Model file for the job. Use its own axes, mm. A direction names the side the tool comes from. Round coordinates to 2 decimals unless told otherwise and drop trailing zeros. Loops run counter-clockwise (first coordinate to the right, second up) from the corner with the lowest first, then second, coordinate; pieces in that order, holes last. Notation, with made-up numbers: (46.25, -2.75) - (99.25, -2.75) arc R24 ccw to (99.25, 24.25) - close; hole circle Ø1 at (60.25, 84). An arc over 180 degrees is marked (long way). Answer as a JSON object with one key per item and string values.
from build123d import *

# Parameters (mm, degrees)
ESQUISSE1_R                  = 18
BOSS_EXTRU_1_DEPTH           = 4
ESQUISSE5_R                  = 25.5
BOSS_EXTRU_2_DEPTH           = 0.6
ENL_V_MAT_EXTRU_1_DEPTH      = 37.354642069
ESQUISSE4_R                  = 4
ENL_V_MAT_EXTRU_3_DEPTH      = 37.354642069
R_P_TITION_CIRCULAIRE1_COUNT = 6
ESQUISSE3_R                  = 3.25
ENL_V_MAT_EXTRU_2_DEPTH      = 37.354642069
R_P_TITION_CIRCULAIRE2_COUNT = 3
CONG_1_R                     = 0.5
ESQUISSE6_R                  = 25.5
ESQUISSE6_R_2                = 23.5
BOSS_EXTRU_3_DEPTH           = 5
ESQUISSE7_W                  = 4
ESQUISSE7_H                  = 4
ENL_V_MAT_EXTRU_4_DEPTH      = 4
R_P_TITION_CIRCULAIRE3_COUNT = 18


with BuildPart() as part:
    # Esquisse1 → Boss.-Extru.1 (new body)
    with BuildSketch(Plane.XY):
        Circle(ESQUISSE1_R)
    extrude(amount=BOSS_EXTRU_1_DEPTH)

    # Esquisse5 → Boss.-Extru.2 (add)
    with BuildSketch(Plane(origin=(0, 0, 0), x_dir=(-1, 0, 0), z_dir=(0, 0, -1))):
        Circle(ESQUISSE5_R)
    extrude(amount=BOSS_EXTRU_2_DEPTH)

    # Esquisse2 → Enl_v. mat.-Extru.1 (cut, through all)
    with BuildSketch(Plane.XY.offset(4)):
        with BuildLine():
            Line((0, 13), (0, 16.5))
            ThreePointArc((0, 16.5), (-4.270514244, 15.937776134), (-8.25, 14.289419162))
            Line((-8.25, 14.289419162), (-6.5, 11.258330249))
            ThreePointArc((-6.5, 11.258330249), (-3.364647586, 12.557035742), (0, 13))
        make_face()
    enl_v_mat_extru_1 = extrude(amount=-ENL_V_MAT_EXTRU_1_DEPTH, mode=Mode.SUBTRACT)

    # Esquisse4 → Enl_v. mat.-Extru.3 (cut, through all)
    with BuildSketch(Plane.XY.offset(4)):
        Circle(ESQUISSE4_R)
    extrude(amount=-ENL_V_MAT_EXTRU_3_DEPTH, mode=Mode.SUBTRACT)

    # R_p_tition circulaire1: Enl_v. mat.-Extru.1 ×6 about axis
    r_p_tition_circulaire1_axis = Axis((0, 0, 0), (0, 0, 1))
    for i in range(1, R_P_TITION_CIRCULAIRE1_COUNT):
        add(enl_v_mat_extru_1.rotate(r_p_tition_circulaire1_axis, i * 360 / R_P_TITION_CIRCULAIRE1_COUNT), mode=Mode.SUBTRACT)

    # Esquisse3 → Enl_v. mat.-Extru.2 (cut, through all)
    with BuildSketch(Plane.XY.offset(4)):
        with Locations((0, 10)):
            Circle(ESQUISSE3_R)
    enl_v_mat_extru_2 = extrude(amount=-ENL_V_MAT_EXTRU_2_DEPTH, mode=Mode.SUBTRACT)

    # R_p_tition circulaire2: Enl_v. mat.-Extru.2 ×3 about axis
    r_p_tition_circulaire2_axis = Axis((0, 0, 0), (0, 0, 1))
    for i in range(1, R_P_TITION_CIRCULAIRE2_COUNT):
        add(enl_v_mat_extru_2.rotate(r_p_tition_circulaire2_axis, i * 360 / R_P_TITION_CIRCULAIRE2_COUNT), mode=Mode.SUBTRACT)

    # Cong_1
    cong_1_edges = [part.edges().sort_by_distance(p)[0] for p in [
        (-1.423076416, 12.921875, 1.7),
        (-10.479133807, -7.693357827, 1.7),
        (11.902210222, -5.228517173, 1.7),
    ]]
    fillet(cong_1_edges, radius=CONG_1_R)

    # Esquisse6 → Boss.-Extru.3 (add)
    with BuildSketch(Plane(origin=(0, 0, -0.6), x_dir=(-1, 0, 0), z_dir=(0, 0, -1))):
        Circle(ESQUISSE6_R)
        Circle(ESQUISSE6_R_2, mode=Mode.SUBTRACT)
    extrude(amount=BOSS_EXTRU_3_DEPTH)

    # Esquisse7 → Enl_v. mat.-Extru.4 (cut)
    with BuildSketch(Plane(origin=(0, 25.5, 0), x_dir=(1, 0, 0), z_dir=(0, 1, 0))):
        with Locations((0, 3.1)):
            Rectangle(ESQUISSE7_W, ESQUISSE7_H)
    enl_v_mat_extru_4 = extrude(amount=-ENL_V_MAT_EXTRU_4_DEPTH, mode=Mode.SUBTRACT)

    # R_p_tition circulaire3: Enl_v. mat.-Extru.4 ×18 about axis
    r_p_tition_circulaire3_axis = Axis((0, 0, 0), (0, 0, 1))
    for i in range(1, R_P_TITION_CIRCULAIRE3_COUNT):
        add(enl_v_mat_extru_4.rotate(r_p_tition_circulaire3_axis, i * 360 / R_P_TITION_CIRCULAIRE3_COUNT), mode=Mode.SUBTRACT)


solid = part.part
1) Slice it at C-C on x = 20. List the corners of the cut face in (y, z).
Values follow:
{"outline": "(-15.82, -5.6) - (-12.34, -5.6) - (-12.34, -5.1) - (-13.86, -5.1) - (-13.86, -1.1) - (-12.34, -1.1) - (-12.34, -0.6) - (12.34, -0.6) - (12.34, -1.1) - (13.86, -1.1) - (13.86, -5.1) - (12.34, -5.1) - (12.34, -5.6) - (15.82, -5.6) - (15.82, 0) - (-15.82, 0) - close"}
2) Slice it at A-A on z = -3.25. Count the separate pieces of the cut face and the enclosed holes in it, then the cut area to 3 significant figures.
Values follow:
{"separate pieces": "18", "enclosed holes": "0", "area": "164 mm²"}
3) Drop flat-ended pins along their axis: P1, Ø1.7, axis at x = 15.5, z = 2.5, coming from the -Y side; P2, Ø3, axis at x = 24.5, y = -4.5, coming from the +Z side; P3, Ø1, axis at x = 4, y = -17.5, coming from the -Z side; P4, Ø4, axis at x = 0, y = 10, coming from the -Z side. Give the stop position or say it passes through.
Values follow:
{"P1": "y = -10.46", "P2": "z = 0", "P3": "z = -0.6", "P4": "through"}
4) Two-plate mould, pull along Y, no slides. Class faces 4 (the flat face through (-20.16, 13.95, -3.07)), 5 (the flat face through (-17.237, -17.431, -3.072)), 6 (the cylindrical face through (4.212, -15.953, 1.732)), 7 (the flat face through (0, 24, -1.1)): pulls with the +Y half, pulls with the -Y half, needs draft (parallel to the pull), parting line crosses it, or undercut.
Values follow:
{"face 4": "undercut", "face 5": "pulls with the -Y half", "face 6": "undercut", "face 7": "needs draft"}
5) Slice it at B-B on y = -5. List the corners of the cut face in (x, z) (3 decimals), then the cut area to 3 significant figures.
Values follow:
{"outline": "(-25.005, -5.6) - (-22.962, -5.6) - (-22.962, -5.1) - (-25.005, -5.1) - close; (-25.005, -1.1) - (-22.962, -1.1) - (-22.962, -0.6) - (-11.91, -0.6) - (-11.91, 4) - (-17.292, 4) - (-17.292, 0) - (-25.005, 0) - close; (-5.41, -0.6) - (5.41, -0.6) - (5.41, 4) - (-5.41, 4) - close; (15.724, -0.6) - (22.962, -0.6) - (22.962, -1.1) - (25.005, -1.1) - (25.005, 0) - (17.292, 0) - (17.292, 4) - (15.724, 4) - close; (22.962, -5.6) - (25.005, -5.6) - (25.005, -5.1) - (22.962, -5.1) - close", "area": "95.1 mm²"}
6) Probe probe 1 along Z at (x, y) = (-21.5, 11.5); probe 2 along Y at (x, z) = (6, 2); probe 3 along X at (y, z) = (-5, 1.05). List the from-to ranges inside material, lowest first.
Values follow:
{"probe 1": "-5.6 to -5.1, -1.1 to 0", "probe 2": "-16.97 to -15.37, -11.53 to -6.87, -3.13 to 16.97", "probe 3": "-17.29 to -11.91, -5.41 to 5.41, 15.72 to 17.29"}
7) Tool access for faces 1 (the flat face through (20.16, -13.95, -3.07)), 2 (the flat face through (-6.477, 23.643, -3.072)), 3 (the flat face through (15, 0, 2)): list every direction of +Z, -Z, +X, -X, +Y, -Y with a clear straight run to the whole face (end or side of a thin tool).
Values follow:
{"face 1": "+X", "face 2": "none", "face 3": "+Z, -Z"}
